Can you work these out from the model? Positions are in its coordinate system, mm. Face numbers are marked on the shaded views. A direction names the side the tool comes from. Give positions to 0.01 mm unless a question says otherwise; leave off trailing zeros. Order: outer loops, then holes, each group sorted by start corner. A loop starts at its lowest first (then second) coordinate and runs counter-clockwise, first axis right, second up. Notation, with made-up numbers: (6, -33) -> (65, -33) arc R16 ccw to (65, -21) -> close; hole circle Ø1 at (53, 42.5). An arc over 180 degrees is marked (long way). Answer as a JSON object with one key per item and string values.
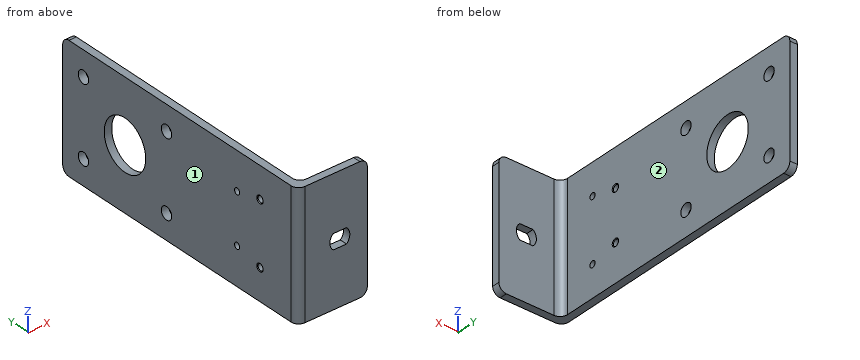
```python
from build123d import *

# Parameters (mm, degrees)
EXTRUDE_THIN1_DEPTH         = 50
HOLE1_D                     = 5
SKETCH3_R                   = 10
CUT_EXTRUDE1_DEPTH          = 125.03225387
M3_TAPPED_HOLE1_D           = 2.5
M3_TAPPED_HOLE1_DEPTH       = 7.5
M3_TAPPED_HOLE1_CSINK_D     = 3.05
M3_TAPPED_HOLE1_CSINK_ANGLE = 90
M3_TAPPED_HOLE1_TIP         = 0.751075774
CUT_EXTRUDE2_DEPTH          = 10
FILLET1_R                   = 3
M3_TAPPED_HOLE2_D           = 2.5
M3_TAPPED_HOLE2_DEPTH       = 7.5
M3_TAPPED_HOLE2_CSINK_D     = 3.05
M3_TAPPED_HOLE2_CSINK_ANGLE = 90
M3_TAPPED_HOLE2_TIP         = 0.751075774
FILLET2_R                   = 3
FILLET3_R                   = 3


with BuildPart() as part:
    # Sketch1 → Extrude-Thin1 (new body)
    with BuildSketch(Plane.XY):
        Polygon((0, 110), (0, 0), (25, 0), (25, -3), (-3, -3), (-3, 110), align=None)
    extrude(amount=EXTRUDE_THIN1_DEPTH)

    # Hole1 (through all)
    with Locations(Plane(origin=(-3, 100, 10), x_dir=(0, -1, 0), z_dir=(-1, 0, 0))):
        with Locations((0, 0), (0, 30), (40, 30), (40, 0)):
            Hole(HOLE1_D / 2)

    # Sketch3 → Cut-Extrude1 (cut, through all)
    with BuildSketch(Plane.ZY.offset(3)):
        with Locations(Location((25, 80, 0), (0, 0, 270))):
            Circle(SKETCH3_R)
    extrude(amount=-CUT_EXTRUDE1_DEPTH, mode=Mode.SUBTRACT)

    # M3 Tapped Hole1
    with Locations(Plane(origin=(-3, 15, 12.5), x_dir=(0, -1, 0), z_dir=(-1, 0, 0))):
        with Locations((0, 0), (0, 25)):
            CounterSinkHole(M3_TAPPED_HOLE1_D / 2, M3_TAPPED_HOLE1_CSINK_D / 2, depth=M3_TAPPED_HOLE1_DEPTH, counter_sink_angle=M3_TAPPED_HOLE1_CSINK_ANGLE)
            with Locations((0, 0, -(M3_TAPPED_HOLE1_DEPTH + M3_TAPPED_HOLE1_TIP / 2))):  # 118° drill point
                Cone(0, M3_TAPPED_HOLE1_D / 2, M3_TAPPED_HOLE1_TIP, mode=Mode.SUBTRACT)

    # Sketch5 → Cut-Extrude2 (cut)
    with BuildSketch(Plane(origin=(0, -3, 0), x_dir=(-1, 0, 0), z_dir=(0, -1, 0))):
        with BuildLine():
            Line((-11.354248689, -22), (-16.645751311, -22))
            ThreePointArc((-16.645751311, -22), (-18, -25), (-16.645751311, -28))
            Line((-16.645751311, -28), (-11.354248689, -28))
            ThreePointArc((-11.354248689, -28), (-10, -25), (-11.354248689, -22))
        make_face()
    extrude(amount=-CUT_EXTRUDE2_DEPTH, mode=Mode.SUBTRACT)

    # Fillet1
    fillet1_edges = [part.edges().sort_by_distance(p)[0] for p in [
        (-1.5, 110, 50),
        (-1.5, 110, 0),
        (25, -1.5, 0),
        (25, -1.5, 50),
    ]]
    fillet(fillet1_edges, radius=FILLET1_R)

    # M3 Tapped Hole2
    with Locations(Plane(origin=(0, 26, 35), x_dir=(0, 1, 0), z_dir=(1, 0, 0))):
        with Locations((0, 0), (0, -20)):
            CounterSinkHole(M3_TAPPED_HOLE2_D / 2, M3_TAPPED_HOLE2_CSINK_D / 2, depth=M3_TAPPED_HOLE2_DEPTH, counter_sink_angle=M3_TAPPED_HOLE2_CSINK_ANGLE)
            with Locations((0, 0, -(M3_TAPPED_HOLE2_DEPTH + M3_TAPPED_HOLE2_TIP / 2))):  # 118° drill point
                Cone(0, M3_TAPPED_HOLE2_D / 2, M3_TAPPED_HOLE2_TIP, mode=Mode.SUBTRACT)

    # Fillet2
    fillet2_edges = [part.edges().sort_by_distance(p)[0] for p in [
        (-3, -3, 25),
    ]]
    fillet(fillet2_edges, radius=FILLET2_R)

    # Fillet3
    fillet3_edges = [part.edges().sort_by_distance(p)[0] for p in [
        (0, 0, 25),
    ]]
    fillet(fillet3_edges, radius=FILLET3_R)


solid = part.part
```
1. If we section it at C-C on x = 15: Please give me the cut outline in (y, z).
Worked answers:
{"outline": "(-3, 0) -> (0, 0) -> (0, 22) -> (-3, 22) -> close; (-3, 28) -> (0, 28) -> (0, 50) -> (-3, 50) -> close"}
2. If we section it at A-A on y = 80: Please give me the cut outline in (x, z).
Worked answers:
{"outline": "(-3, 0) -> (0, 0) -> (0, 15) -> (-3, 15) -> close; (-3, 35) -> (0, 35) -> (0, 50) -> (-3, 50) -> close"}
3. If we section it at D-D on y = 15: Please give me the cut outline in (x, z) (3 decimals), then the cut area to 3 significant figures.
Worked answers:
{"outline": "(-3, 0) -> (0, 0) -> (0, 11.25) -> (-2.725, 11.25) -> (-3, 10.975) -> close; (-3, 14.025) -> (-2.725, 13.75) -> (0, 13.75) -> (0, 36.25) -> (-2.725, 36.25) -> (-3, 35.975) -> close; (-3, 39.025) -> (-2.725, 38.75) -> (0, 38.75) -> (0, 50) -> (-3, 50) -> close", "area": "135 mm²"}
4. If we section it at B-B on z = 25: Please give me the cut outline in (x, y), then the cut area to 3 significant figures.
Worked answers:
{"outline": "(-3, 0) arc R3 ccw to (0, -3) -> (10, -3) -> (10, 0) -> (3, 0) arc R3 cw to (0, 3) -> (0, 70) -> (-3, 70) -> close; (-3, 90) -> (0, 90) -> (0, 110) -> (-3, 110) -> close; (18, -3) -> (25, -3) -> (25, 0) -> (18, 0) -> close", "area": "330 mm²"}
5. For the marked faces 1 and 2, which set-ups out of +Z, -Z, +X, -X, +Y, -Y let a thin tool reach every point of the face, with its end or its side?
Worked answers:
{"face 1": "+Z, -Z, -X, +Y, -Y", "face 2": "+Z, -Z, +X, +Y"}
6. Will these pins go through, and if not, where does the flat tip stop? pin 1 Ø1 at (y, z) = (79.5, 10.5) entering from +X; pin 2 Ø2 at (x, y) = (1.5, 31.5) entering from +Z; pin 3 Ø6 at (y, z) = (100, 10) entering from -X; pin 4 Ø11 at (x, z) = (12.5, 28) entering from +Y.
Worked answers:
{"pin 1": "x = 0", "pin 2": "through", "pin 3": "x = -3", "pin 4": "y = 0"}
7. Please list where these lines run through material, in increasing order: L1, parallel to Z at x = -0.65, y = 100; L2, parallel to Z at x = -1, y = 60.5; L3, parallel to X at y = 95.5, z = 29.
Worked answers:
{"L1": "0 to 7.5, 12.5 to 37.5, 42.5 to 50", "L2": "0 to 7.55, 12.45 to 37.55, 42.45 to 50", "L3": "-3 to 0"}
